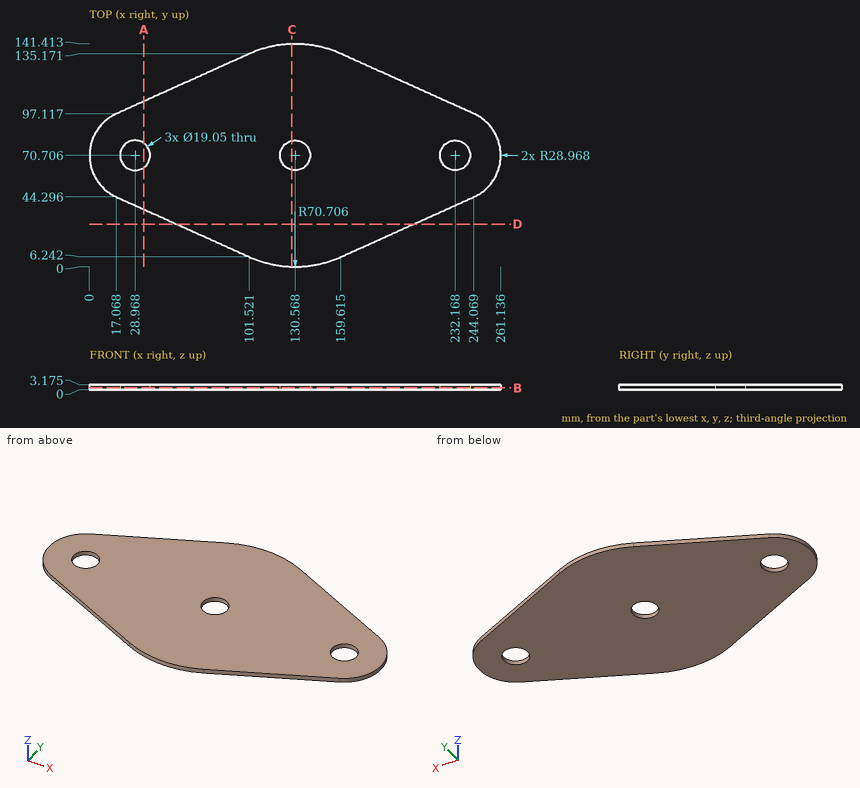
Can you work these out from the drawing? Everything is in mm from the part's minimum corner. Coordinates: 2 decimals unless noted, no trailing zeros. Loops run counter-clockwise (first coordinate to the right, second up) from the corner with the lowest first, then second, coordinate; pieces in that order, holes last.
1. Imagine slicing it at C-C, the plane x = 128.5. Please give me the cut outline in (y, z) (1 decimal).
2. For P1, Ø17, axis at x = 28.97, y = 70.71, coming from the -Z side; P2, Ø1.5, axis at y = 24, z = 2, coming from the +X side, each with a flat end and sliding along its axis, tell me the tip position at first contact or that it passes through.
3. Imagine slicing it at A-A, the plane x = 34.5. Please give me the cut outline in (y, z) (1 decimal).
4. Imagine slicing it at D-D, the plane y = 27. Please give me the cut outline in (x, z) (1 decimal).
5. Imagine slicing it at B-B, the plane z = 1.2. Count the separate pieces of the cut face and the enclosed holes in it, and give its area (3 significant figures).
6. I need wall thicknesses on L1, parallel to Y at x = 130.5, z = 1.7; L2, parallel to X at y = 77, z = 1.6 (1 decimal); L3, parallel to Y at x = 34, z = 0.7 (1 decimal). Which ranges of each line are inside material? Lowest first, please.
Taken from the geometry:
1. outline: (0, 0) - (61.4, 0) - (61.4, 3.2) - (0, 3.2) - close; (80, 0) - (141.4, 0) - (141.4, 3.2) - (80, 3.2) - close
2. P1: passes through
2. P2: stops at x = 200.69
3. outline: (36.4, 0) - (63, 0) - (63, 3.2) - (36.4, 3.2) - close; (78.5, 0) - (105, 0) - (105, 3.2) - (78.5, 3.2) - close
4. outline: (55.5, 0) - (205.7, 0) - (205.7, 3.2) - (55.5, 3.2) - close
5. separate pieces: 1
5. enclosed holes: 3
5. area: 23,800 mm2
6. L1: y = 0 to 61.18, 80.23 to 141.41
6. L2: x = 0.7 to 21.8, 36.1 to 123.4, 137.7 to 225, 239.3 to 260.4
6. L3: y = 36.7 to 62.6, 78.8 to 104.7
